Autodesk Fusion 360 part; units mm, degrees
sketch "Sketch1" plane through (0, 0, 0) normal (0, 1, 0) x (1, 0, 0)
  circle A0 centre (0, 0) radius 8.5
  circle A1 centre (0, 0) radius 9.5
  circle A2 centre (0, 0) radius 4.25
  dimension "d1" = 17
  dimension "d2" = 19
  dimension "d7" = 8.5
extrude "Extrude1" add sketch "Sketch1" along normal blind 20 contours A1
extrude "Extrude2" add sketch "Sketch1" along normal blind 20 contours A0 | A2
extrude "Extrude3" cut sketch "Sketch1" along normal blind 20 contours A2
extrude "Extrude4" cut 1 faces at (7.7146, 20, 0.472) along direction (0, -1, 0) blind 10
extrude "Extrude5" cut sketch "Sketch1" along normal blind 4 contours A0
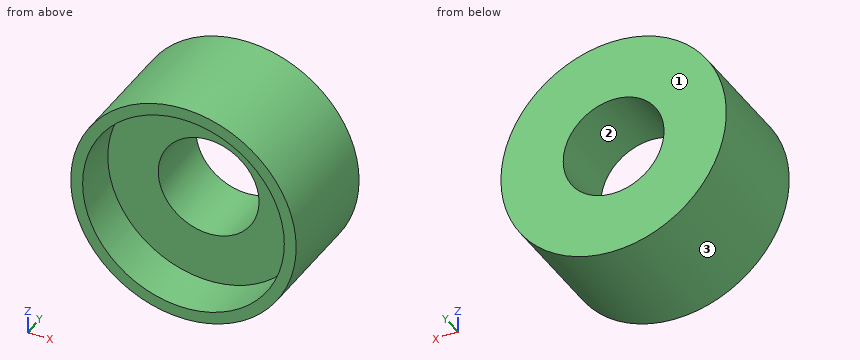
Input: part model. Units: mm. Frame: model coordinates. Face numbers are marked on the shaded views. Round coordinates to 2 decimals unless told otherwise and drop trailing zeros. Loops run counter-clockwise (first coordinate to the right, second up) from the corner with the lowest first, then second, coordinate; pieces in that order, holes last. Notation, with made-up numbers: (41, 0) -> (76, 0) arc R21 ccw to (76, 26) -> close; hole circle Ø9 at (89, 28). An arc over 180 degrees is marked (long way). Answer as a JSON object with one key per item and string values. Group by question number.
1) Ray query, L1, parallel to Z at x = 0, y = 6.6; L2, parallel to Z at x = 0, y = 1.3; L3, parallel to Y at x = 0, z = -6.75. Return the intervals inside material, ascending.
2) Draft query along X for the marked faces 1, 2 and 3. Return one class per face: +X half, -X half, draft (parallel to the pull), parting line (faces both ways), or undercut.
3) Section query B-B on z = 0. Output: boundary loops of the cut face in (x, y), plus the area to 3 significant figures.
4) Section query D-D on x = -4.5. Output: boundary loops of the cut face in (y, z).
5) Pin query (flat end, axial travel): pin 1 (1 mm diameter, centred on y = 1, z = -2.5, fed in from +X); pin 2 (1.5 mm diameter, centred on y = 8, z = 2.5, fed in from -X); pin 3 (1 mm diameter, centred on x = -2, z = -6.5, fed in from -Y). Return the tip coordinate at first contact, or that it passes through.
6) Section query C-C on y = 1.5. Output: boundary loops of the cut face in (x, z), plus the area to 3 significant figures.
7) Section query A-A on x = 0. Output: boundary loops of the cut face in (y, z).
Reply:
{
 "1": {"L1": "z = -9.5 to -4.25, 4.25 to 9.5", "L2": "z = -9.5 to -8.5, 8.5 to 9.5", "L3": "y = 4 to 10"},
 "2": {"face 1": "draft", "face 2": "undercut", "face 3": "parting line"},
 "3": {"outline": "(-9.5, 0) -> (-8.5, 0) -> (-8.5, 4) -> (-4.25, 4) -> (-4.25, 10) -> (-9.5, 10) -> close; (4.25, 4) -> (8.5, 4) -> (8.5, 0) -> (9.5, 0) -> (9.5, 10) -> (4.25, 10) -> close", "area": "71.0 mm2"},
 "4": {"outline": "(0, -8.37) -> (10, -8.37) -> (10, 8.37) -> (0, 8.37) -> (0, 7.21) -> (4, 7.21) -> (4, -7.21) -> (0, -7.21) -> close"},
 "5": {"pin 1": "stops at x = 9.29", "pin 2": "stops at x = -9.34", "pin 3": "stops at y = 4"},
 "6": {"outline": "circle Ø19 at (0, 0); hole circle Ø17 at (0, 0)", "area": "56.5 mm2"},
 "7": {"outline": "(0, -9.5) -> (10, -9.5) -> (10, -4.25) -> (4, -4.25) -> (4, -8.5) -> (0, -8.5) -> close; (0, 8.5) -> (4, 8.5) -> (4, 4.25) -> (10, 4.25) -> (10, 9.5) -> (0, 9.5) -> close"}
}
